Geometry check sheet. Reference: drawing and pictorial views, mm from the part's lowest x, y, z. A direction names the side the tool comes from. Round coordinates to 2 decimals unless told otherwise and drop trailing zeros. Write each loop counter-clockwise with the first axis right and the second up, starting at its lowest first coordinate (ties: lowest second). Pieces come first, ordered by that corner, then holes. Notation, with made-up numbers: M 22.5,15.25 L 59.5,15.25 A22 ccw 59.5,31.25 Z; hole C 53.5,24.25 d2. An arc over 180 degrees is marked long. Put each result on its own line as item: value. Start each with the question number.
(1) Section check A-A on y = 20. Record the cut outline in (x, z), then the cut area to 3 significant figures.
(2) Section check C-C on z = 7. Record the cut outline in (x, y).
(3) Section check D-D on x = 23. Record the cut outline in (y, z), then the cut area to 3 significant figures.
(4) Gauge pin test, flat ends, axial feed: pin 1 (8 mm diameter, centred on x = 12, y = 8, fed in from -Z); pin 2 (2 mm diameter, centred on x = 18.5, z = 9, fed in from +Y); pin 3 (2.5 mm diameter, centred on x = 39.5, z = 7, fed in from +Y). Record the tip position at first contact, or that the pin passes through.
(5) Section check B-B on x = 15. Record the cut outline in (y, z), then the cut area to 3 significant figures.
(6) Tool access check on the marked faces 1 and 2. Record the directions out of +Z, -Z, +X, -X, +Y, -Y that give a thin tool (end or side, any length) a straight path to the whole face; none if there is none.
(7) Material ranges on probe 1 along X at (y, z) = (1.85, 25); probe 2 along X at (y, z) = (2.1, 16); probe 3 along Z at (x, y) = (15, 2.45), recorded low to high.
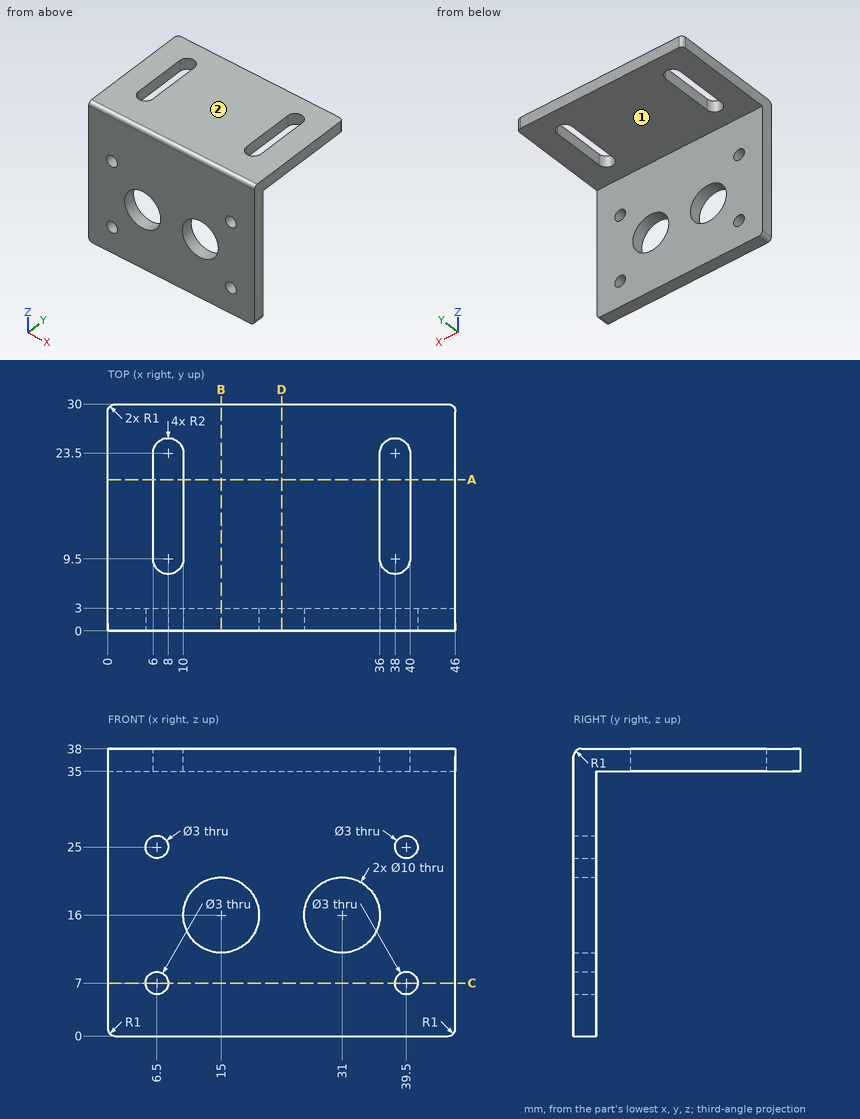
Answers follow:
1. outline: M 0,35 L 6,35 L 6,38 L 0,38 Z; M 10,35 L 36,35 L 36,38 L 10,38 Z; M 40,35 L 46,35 L 46,38 L 40,38 Z
1. area: 114 mm^2
2. outline: M 0,0 L 5,0 L 5,3 L 0,3 Z; M 8,0 L 38,0 L 38,3 L 8,3 Z; M 41,0 L 46,0 L 46,3 L 41,3 Z
3. outline: M 0,0 L 3,0 L 3,35 L 30,35 L 30,38 L 1,38 A1 ccw 0,37 Z
3. area: 195 mm^2
4. pin 1: stops at z = 35
4. pin 2: stops at y = 3
4. pin 3: passes through
5. outline: M 0,0 L 3,0 L 3,11 L 0,11 Z; M 0,21 L 3,21 L 3,35 L 30,35 L 30,38 L 1,38 A1 ccw 0,37 Z
5. area: 165 mm^2
6. face 1: -Z, +X, -X, +Y
6. face 2: +Z, +X, -X, +Y, -Y
7. probe 1: x = 0 to 5, 8 to 38, 41 to 46
7. probe 2: x = 0 to 10, 20 to 26, 36 to 46
7. probe 3: z = 0 to 11, 21 to 38
